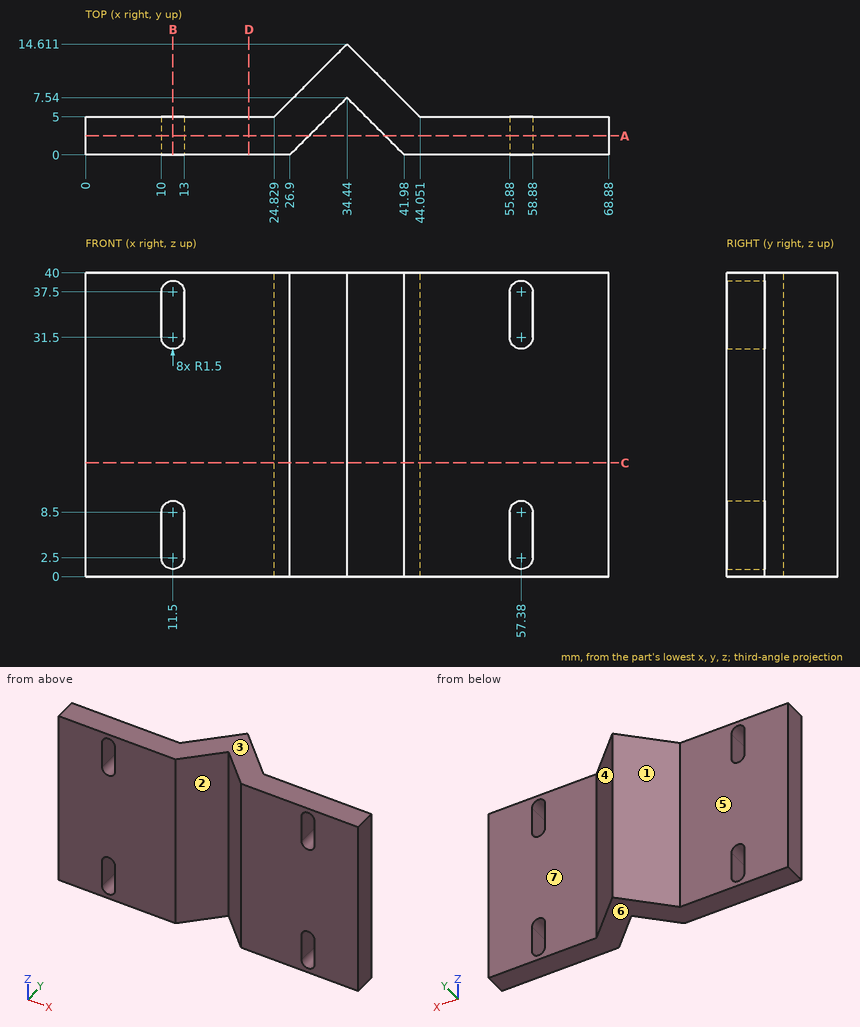
Design review of the part shown in the three views and the two pictorial views. Dimensions are in mm from the part's minimum x, y and z. A direction names the side the tool comes from. Give positions to 0.01 mm unless a question says otherwise; leave off trailing zeros. Order: outer loops, then holes, each group sorted by start corner. A loop starts at its lowest first (then second) coordinate and runs counter-clockwise, first axis right, second up. Notation, with made-up numbers: (1, 7.25) -> (54, 7.25) arc R18 ccw to (54, 20.25) -> close; hole circle Ø3 at (-11, 87). An arc over 180 degrees is marked (long way). Write each question's results on one line, items separated by ' | '. Start each with the question number.
Q1. Mouldability with a two-part tool opening along X and no side actions: class the marked faces 1, 2, 3 and 4 as +X half, -X half, draft (parallel to the pull), parting line (faces both ways), or undercut.
Q2. Wall thickness on L1, parallel to Y at x = 19, z = 25; L2, parallel to X at y = 3.5, z = 26; L3, parallel to X at y = 5.75, z = 19.5: over which ranges is each line inside the solid? List them lowest first. Write a range as from..to.
Q3. Add section A-A on y = 2.5. Give the boundary of the cut face in (x, z).
Q4. Add section D-D on x = 21.5. Give the boundary of the cut face in (y, z).
Q5. Add section B-B on x = 11.5. Give the boundary of the cut face in (y, z).
Q6. For pin 1 (1 mm diameter, centred on x = 36.5, z = 19.5, fed in from -Y); pin 2 (1.5 mm diameter, centred on y = 11.5, z = 14.5, fed in from -X); pin 3 (1.5 mm diameter, centred on x = 25, z = 11, fed in from +Y), all flat-tipped, find the tip position at first contact; note any pin that passes through.
Q7. Add section C-C on z = 15. Give the boundary of the cut face in (x, y), and give its area (3 significant figures).
Q8. Machinability: for the marked faces 5, 6 and 7, which of the approach directions +Z, -Z, +X, -X, +Y, -Y give a long, thin tool a straight path to every point of the face, cutting with its end or side? Answer none if there is none.
Found:
1) face 1: -X half | face 2: undercut | face 3: draft | face 4: +X half
2) L1: y = 0..5 | L2: x = 0..30.4, 38.48..68.88 | L3: x = 25.58..32.65, 36.23..43.3
3) outline: (0, 0) -> (29.4, 0) -> (29.4, 40) -> (0, 40) -> close; (39.48, 0) -> (68.88, 0) -> (68.88, 40) -> (39.48, 40) -> close; hole (10, 2.5) arc R1.5 ccw to (13, 2.5) -> (13, 8.5) arc R1.5 ccw to (10, 8.5) -> close; hole (10, 31.5) arc R1.5 ccw to (13, 31.5) -> (13, 37.5) arc R1.5 ccw to (10, 37.5) -> close; hole (55.88, 2.5) arc R1.5 ccw to (58.88, 2.5) -> (58.88, 8.5) arc R1.5 ccw to (55.88, 8.5) -> close; hole (55.88, 31.5) arc R1.5 ccw to (58.88, 31.5) -> (58.88, 37.5) arc R1.5 ccw to (55.88, 37.5) -> close
4) outline: (0, 0) -> (5, 0) -> (5, 40) -> (0, 40) -> close
5) outline: (0, 0) -> (5, 0) -> (5, 1) -> (0, 1) -> close; (0, 10) -> (5, 10) -> (5, 30) -> (0, 30) -> close; (0, 39) -> (5, 39) -> (5, 40) -> (0, 40) -> close
6) pin 1: stops at y = 4.98 | pin 2: stops at x = 30.58 | pin 3: stops at y = 5.92
7) outline: (0, 0) -> (26.9, 0) -> (34.44, 7.54) -> (41.98, 0) -> (68.88, 0) -> (68.88, 5) -> (44.05, 5) -> (34.44, 14.61) -> (24.83, 5) -> (0, 5) -> close | area: 380 mm2
8) face 5: +Z, -Z, -X, +Y | face 6: -Z, +X, -X, +Y, -Y | face 7: +Z, -Z, +X, +Y
